from build123d import *

# Parameters (mm, degrees)
SKETCH1_W           = 200
SKETCH1_H           = 100
BOSS_EXTRUDE1_DEPTH = 5
SKETCH2_R           = 2.05
BOSS_EXTRUDE2_DEPTH = 10
SKETCH3_R           = 5
CUT_EXTRUDE1_DEPTH  = 10


with BuildPart() as part:
    # Sketch1 → Boss-Extrude1 (new body)
    with BuildSketch(Plane(origin=(0, 0, 0), x_dir=(1, 0, 0), z_dir=(0, 1, 0))):
        with Locations((100, 50)):
            Rectangle(SKETCH1_W, SKETCH1_H)
    extrude(amount=BOSS_EXTRUDE1_DEPTH)

    # Sketch2 → Boss-Extrude2 (add)
    with BuildSketch(Plane(origin=(0, 5, 0), x_dir=(1, 0, 0), z_dir=(0, 1, 0))):
        with Locations((2.5, 97.5)):
            Circle(SKETCH2_R)
        with Locations((197.5, 97.5)):
            Circle(SKETCH2_R)
        with Locations((197.5, 2.5)):
            Circle(SKETCH2_R)
        with Locations((2.5, 2.5)):
            Circle(SKETCH2_R)
        with Locations((67.5, 50)):
            Circle(SKETCH2_R)
        with Locations((132.5, 50)):
            Circle(SKETCH2_R)
    extrude(amount=BOSS_EXTRUDE2_DEPTH)

    # Sketch3 → Cut-Extrude1 (cut)
    with BuildSketch(Plane(origin=(0, 0, 0), x_dir=(-1, 0, 0), z_dir=(0, -1, 0))):
        with Locations((-170, 70)):
            Circle(SKETCH3_R)
        with Locations((-30, 70)):
            Circle(SKETCH3_R)
    extrude(amount=-CUT_EXTRUDE1_DEPTH, mode=Mode.SUBTRACT)


solid = part.part
Source: CAD feature listing. Evaluate the final solid. Frame: model axes, mm. A direction names the side the tool comes from. Coordinates: 2 decimals unless noted, no trailing zeros. Write each loop counter-clockwise with the first axis right and the second up, starting at its lowest first coordinate (ties: lowest second). Pieces come first, ordered by that corner, then holes. Notation, with made-up numbers: M 75,-33.5 L 88,-33.5 A18 ccw 88,-15.5 Z; hole C 86,8.25 d9. An arc over 180 degrees is marked long. Use a Markdown table: item, result.
1) Section C-C, the plane y = 8.75. Output: boundary loops of the cut face in (x, z), then the cut area to 3 significant figures.
Conclusion:
| item | result |
|---|---|
| outline | C 2.5,-97.5 d4.1; C 2.5,-2.5 d4.1; C 67.5,-50 d4.1; C 132.5,-50 d4.1; C 197.5,-97.5 d4.1; C 197.5,-2.5 d4.1 |
| area | 79.2 mm^2 |
2) Ray query, L1, parallel to X at y = 2.65, z = -70; L2, parallel to Z at x = 30, y = 3.9; L3, parallel to Y at x = 70.5, z = -61.5. Return the intervals inside material, ascending.
Conclusion:
| item | result |
|---|---|
| L1 | x = 0 to 25, 35 to 165, 175 to 200 |
| L2 | z = -100 to -75, -65 to 0 |
| L3 | y = 0 to 5 |
3) Mould query, pull axis X, two halves, no side actions, for faces 1 (the flat face through (99, 2, 0)), 2 (the cylindrical face through (134.455, 9.93, -50.616)), 3 (the flat face through (0, 2, -49)). Classes: pulls with the +X half, pulls with the -X half, needs draft (parallel to the pull), parting line crosses it, or undercut.
Conclusion:
| item | result |
|---|---|
| face 1 | needs draft |
| face 2 | undercut |
| face 3 | pulls with the -X half |
4) First-contact query: pin 1 Ø5 at (x, y) = (52.5, 9) entering from +Z; pin 2 Ø6 at (x, z) = (124, -47) entering from +Y; pin 3 Ø8 at (x, y) = (62, 10) entering from +Z. Flat tips, straight axial feed; report the tip coordinate or a pass-through.
Conclusion:
| item | result |
|---|---|
| pin 1 | passes through |
| pin 2 | stops at y = 5 |
| pin 3 | stops at z = -48.6 |
5) Section B-B, the plane x = 197.5. Output: boundary loops of the cut face in (y, z).
Conclusion:
| item | result |
|---|---|
| outline | M 0,-100 L 5,-100 L 5,-99.55 L 15,-99.55 L 15,-95.45 L 5,-95.45 L 5,-4.55 L 15,-4.55 L 15,-0.45 L 5,-0.45 L 5,0 L 0,0 Z |
6) Section D-D, the plane x = 67.5. Output: boundary loops of the cut face in (y, z).
Conclusion:
| item | result |
|---|---|
| outline | M 0,-100 L 5,-100 L 5,-52.05 L 15,-52.05 L 15,-47.95 L 5,-47.95 L 5,0 L 0,0 Z |
7) Reachability of faces 4 (the cylindrical face through (199.455, 9.93, -98.116)), 5 (the flat face through (99, 2, -100)) from +Z, -Z, +X, -X, +Y, -Y: full face, straight path, thin tool, end or side. Return the list, or none.
Conclusion:
| item | result |
|---|---|
| face 4 | +Y |
| face 5 | -Z, +X, -X, +Y, -Y |
8) Section A-A, the plane z = -50. Output: boundary loops of the cut face in (x, y), then the cut area to 3 significant figures.
Conclusion:
| item | result |
|---|---|
| outline | M 0,0 L 200,0 L 200,5 L 134.55,5 L 134.55,15 L 130.45,15 L 130.45,5 L 69.55,5 L 69.55,15 L 65.45,15 L 65.45,5 L 0,5 Z |
| area | 1,080 mm^2 |
